Build history of the part. All positions in model axes, mm. Round coordinates to 2 decimals unless told otherwise and drop trailing zeros. Write each loop counter-clockwise with the first axis right and the second up, starting at its lowest first coordinate (ties: lowest second). Pieces come first, ordered by that corner, then holes. Notation, with made-up numbers: (89.5, 21.25) -> (97.5, 21.25) arc R15 cw to (97.5, 30.25) -> close; hole circle Ø8 at (34.5, 15.25). An arc over 180 degrees is marked (long way). Return JSON: item names as keys, results as strings.
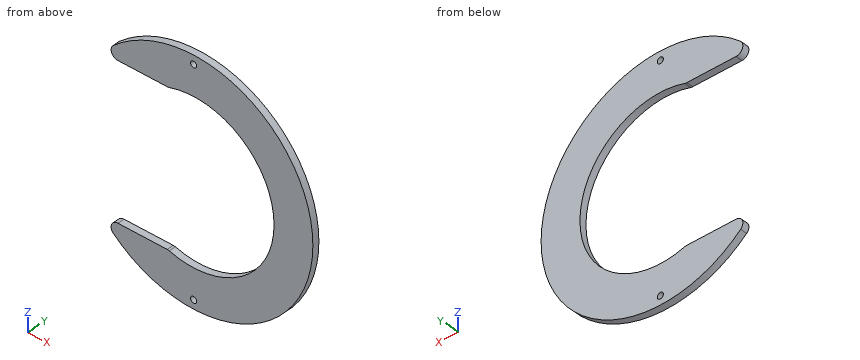
Autodesk Inventor part; units mm, degrees
ref_plane "YZ Plane" through (0, 0, 0) normal (1, 0, 0) x (0, 1, 0)
ref_plane "XZ Plane" through (0, 0, 0) normal (0, 1, 0) x (-1, 0, 0)
ref_plane "XY Plane" through (0, 0, 0) normal (0, 0, 1) x (1, 0, 0)
sketch "Sketch1" plane through (0, 0, 0) normal (0, 1, 0) x (-1, 0, 0)
  circle A0 centre (0, 0) radius 59
  circle A1 centre (0, 0) radius 81
  circle A2 centre (0, 0) radius 87.5
  circle A3 centre (0, 81) radius 2.25
  circle A4 centre (0, -81) radius 2.25
  line L0 (90, -56) -> (15, -56)
  line L1 (10, -51) -> (10, 51)
  line L2 (15, 56) -> (90, 56)
  line L3 (90, 56) -> (90, -56)
  line L4 (90, -56) -> (10, 56) construction
  line L5 (10, -56) -> (90, 56) construction
  arc A5 (10, -51) -> (15, -56) centre (15, -51) ccw
  arc A6 (15, 56) -> (10, 51) centre (15, 51) ccw
  point P0 (50, 0)
  point P1 (90, 0)
  point P2 (10, 0)
  point P3 (60, -54.4151)
  point P4 (60, 54.4151)
  point P5 (80, 35.4436)
  point P6 (80, -35.4436)
  point P7 (67.2328, 56)
  point P8 (67.2328, -56)
  dimension "d0" = 118
  dimension "d1" = 162
  dimension "d2" = 175
  dimension "d3" = 4.5
  dimension "d4" = 4.5
  dimension "d7" = 112
  dimension "d9" = 80
  dimension "d10" = 10
  dimension "d11" = 5
extrude "Extrusion1" add sketch "Sketch1" along normal blind 5 contours A0 L0 A1 A4 A3 L2 | A1 A3 A4 L0 A2 L2
fillet "Fillet1" radius 5 4 edges at (-67.2328, 2.5, -56) (-67.2328, 2.5, 56) (-18.5742, 2.5, -56) (-18.5742, 2.5, 56)
properties part number "Cylinder Segment Holder"
Q1. Wall check: L1, parallel to Z at x = 0, y = 2.6; L2, parallel to Z at x = 38.5, y = 1.45; L3, parallel to X at y = 3.75, z = -81. Give the ranges that are in metal, low to high.
Verdict:
{"L1": "z = -87.5 to -83.25, -78.75 to -59, 59 to 78.75, 83.25 to 87.5", "L2": "z = -78.57 to -44.71, 44.71 to 78.57", "L3": "x = -33.09 to -2.25, 2.25 to 33.09"}
Q2. Saw through at B-B on z = -81. List the corners of the cut face in (x, y), then the cut area to 3 significant figures.
Verdict:
{"outline": "(-33.09, 0) -> (-2.25, 0) -> (-2.25, 5) -> (-33.09, 5) -> close; (2.25, 0) -> (33.09, 0) -> (33.09, 5) -> (2.25, 5) -> close", "area": "308 mm²"}
Q3. Saw through at D-D on z = 0. List the corners of the cut face in (x, y), then the cut area to 4 significant figures.
Verdict:
{"outline": "(59, 0) -> (87.5, 0) -> (87.5, 5) -> (59, 5) -> close", "area": "142.5 mm²"}
Q4. Pin check, flat tips, straight feed: pin 1 Ø7 at (x, z) = (0, 81) entering from +Y; pin 2 Ø1.5 at (x, y) = (-34.5, 3.5) entering from +Z; pin 3 Ø3 at (y, z) = (2.5, 39) entering from +X; pin 4 Ø3.5 at (x, z) = (0, -81) entering from +Y. Stop position of each tip, or through.
Verdict:
{"pin 1": "stops at y = 5", "pin 2": "stops at z = 80.73", "pin 3": "stops at x = 79.06", "pin 4": "passes through"}
Q5. Saw through at C-C on x = 49.5. List the corners of the cut face in (y, z), then the cut area to 3 significant figures.
Verdict:
{"outline": "(0, -72.15) -> (5, -72.15) -> (5, -32.11) -> (0, -32.11) -> close; (0, 32.11) -> (5, 32.11) -> (5, 72.15) -> (0, 72.15) -> close", "area": "400 mm²"}
Q6. Saw through at A-A on y = 2.95. List the corners of the cut face in (x, z).
Verdict:
{"outline": "(-58.91, -64.7) arc R87.5 ccw (long way) to (-58.91, 64.7) arc R5 ccw to (-55.55, 56) -> (-19.36, 56) arc R5 ccw to (-17.85, 56.23) arc R59 cw (long way) to (-17.85, -56.23) arc R5 ccw to (-19.36, -56) -> (-55.55, -56) arc R5 ccw to start; hole circle Ø4.5 at (0, -81); hole circle Ø4.5 at (0, 81)"}
